from build123d import *

# Parameters (mm, degrees)
F0_W     = 25.4
F0_H     = 50.8
F1_DEPTH = 12.7
F2_SIZE  = 12.69999
F3_R     = 6.35
F4_DEPTH = 25.401


# Not quite as in the source:
# - a fillet or chamfer is up to 0.001 mm smaller than in the source, because OpenCascade refuses the exact size


with BuildPart() as f1:
    # F0 (on Top) → F1 (new body, symmetric)
    with BuildSketch(Plane.XY):
        Polygon((-12.7, -29.3496451829), (-38.1, -29.3496451829), (-38.1, -816.7496451829), (0, -937.8999237629), (38.1, -816.7496451829), (38.1, -29.3496451829), (12.7, -29.3496451829), align=None)
        with Locations((0, -3.9496451829)):
            Rectangle(F0_W, F0_H)
    extrude(amount=F1_DEPTH, both=True)

    # F2 (size 12.7 in the source; OpenCascade refuses exactly that, so slightly less here)
    f2_edges = [f1.edges().sort_by_distance(p)[0] for p in [
        (38.1, -423.049645, 12.7),
        (19.05, -877.324784, 12.7),
        (-19.05, -877.324784, 12.7),
        (-38.1, -423.049645, 12.7),
        (19.05, -877.324784, -12.7),
        (-38.1, -423.049645, -12.7),
        (-19.05, -877.324784, -12.7),
        (38.1, -423.049645, -12.7),
    ]]
    chamfer(f2_edges, length=F2_SIZE)

    # F3 (on face) → F4 (cut, through all)
    with BuildSketch(Plane.XY.offset(12.7)):
        with Locations((0, 8.7503548171)):
            Circle(F3_R)
        with Locations((0, -16.6496451829)):
            Circle(F3_R)
    extrude(amount=-F4_DEPTH, mode=Mode.SUBTRACT)


solid = f1.part
The listing builds one solid part. Answer for the finished solid, in the listing's coordinates (mm). A direction names the side the tool comes from. Give positions to 0.01 mm unless a question says otherwise; leave off trailing zeros. Write each loop counter-clockwise with the first axis right and the second up, starting at its lowest first coordinate (ties: lowest second). Pieces come first, ordered by that corner, then holes. Notation, with made-up numbers: (83, 23.5) - (110, 23.5) arc R21 cw to (110, 53.5) - close; hole circle Ø5 at (-29.75, 61). An arc over 180 degrees is marked (long way). One line per question, with ' | ' between items. Start each with the question number.
1. Straight lines are drawn through the part: line 1 (X direction, y = -239, z = -9); line 2 (X direction, y = -702, z = -4.5); line 3 (Z direction, x = 33, y = -471). For each, find the intervals that lie inside material, in ascending order.
2. For faces 1 (the face through (-12.7, -4, 0)), 2 (the face through (-17.41, -861.08, -6.44)), 3 (the face through (12.7, -4, 0)), determine the directions among +Z, -Z, +X, -X, +Y, -Y from which every point of the face is accessible in a straight line to the end or side of a thin tool.
3. Determine the mould class of faces 4 (the face through (0, -431, -12.7)), 5 (the face through (-17.58, -861.14, 6.26)), 6 (the face through (23, -29.35, 0)) for opening direction Z: +Z half, -Z half, draft (parallel to the pull), parting line (faces both ways), or undercut.
4. Section A-A, the plane z = 7.25 is taken. Determine the outline of the cut face in (x, y).
5. Given P1, Ø7.5, axis at y = 8.5, z = -5.5, coming from the -X side; P2, Ø5, axis at y = -384.5, z = 8, coming from the +X side; P3, Ø8, axis at x = 30.5, z = -7, coming from the +Y side, each flat-ended and moving along its own axis, determine where each tip first touches the part or whether it passes through.
Result:
1) line 1: x = -29.1 to 29.1 | line 2: x = -33.6 to 33.6 | line 3: z = -5.1 to 5.1
2) face 1: +Z, -Z, -X, +Y | face 2: -Z, -X, -Y | face 3: +Z, -Z, +X, +Y
3) face 4: -Z half | face 5: +Z half | face 6: draft
4) outline: (-30.85, -815.64) - (0, -913.73) - (30.85, -815.64) - (30.85, -29.35) - (12.7, -29.35) - (12.7, 21.45) - (-12.7, 21.45) - (-12.7, -29.35) - (-30.85, -29.35) - close; hole circle Ø12.7 at (0, -16.65); hole circle Ø12.7 at (0, 8.75)
5) P1: stops at x = -12.7 | P2: stops at x = 32.6 | P3: stops at y = -29.35
